Job drawing, mm, ordinate dimensions from the low corner. One solid piece. Give positions to 0.01 mm unless a question says otherwise; leave off trailing zeros. Loops run counter-clockwise (first coordinate to the right, second up) from the corner with the lowest first, then second, coordinate; pieces in that order, holes last. Notation, with made-up numbers: M 66,15 L 115,15 A21 ccw 115,22 Z; hole C 26,50.5 d8. An arc over 180 degrees is marked long. One line per question, with ' | ' between items.
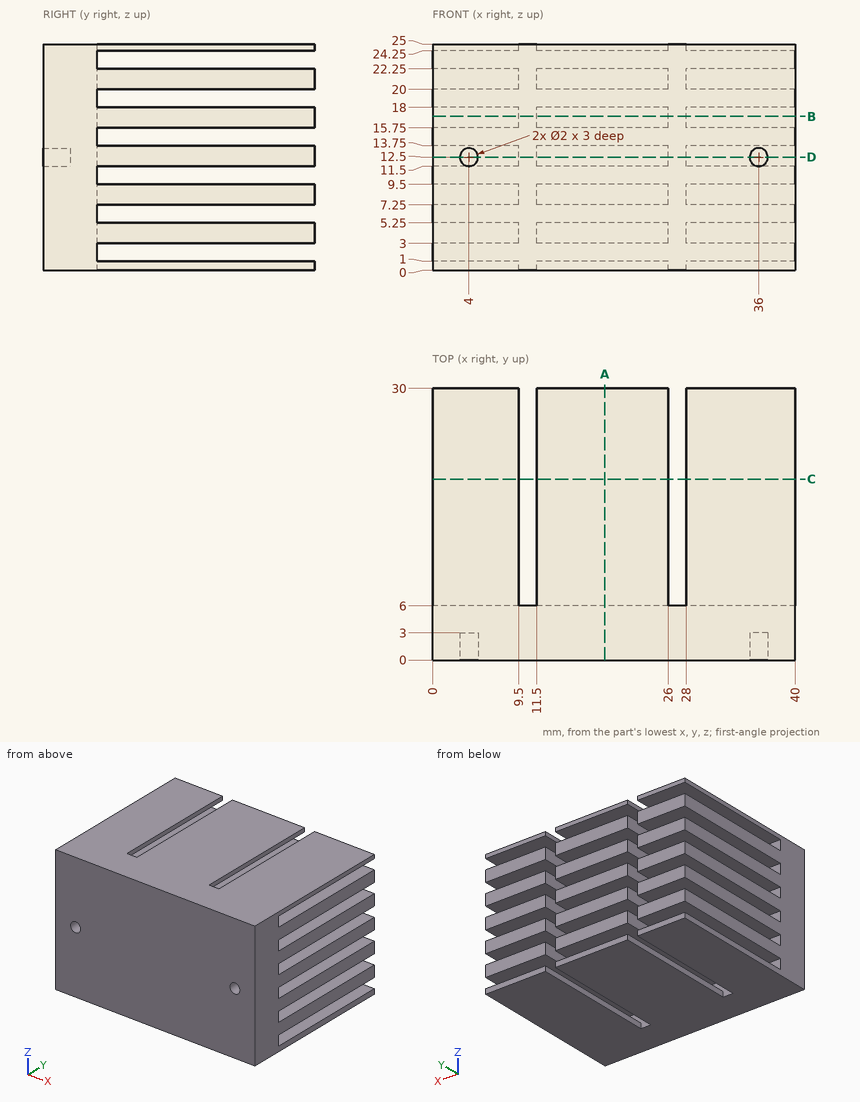
Item 1: Saw through at C-C on y = 20. State how many separate pieces and enclosed holes the cut face has, and give its area (3 significant figures).
Conclusion:
separate pieces: 21 | enclosed holes: 0 | area: 468 mm²
Item 2: Saw through at D-D on z = 12.5. Give the cut face in (x, y), and give its area (3 significant figures).
Conclusion:
outline: M 0,0 L 3,0 L 3,3 L 5,3 L 5,0 L 35,0 L 35,3 L 37,3 L 37,0 L 40,0 L 40,30 L 28,30 L 28,6 L 26,6 L 26,30 L 11.5,30 L 11.5,6 L 9.5,6 L 9.5,30 L 0,30 Z | area: 1,090 mm²
Item 3: Saw through at A-A on x = 19. Give the cut face in (y, z).
Conclusion:
outline: M 0,0 L 30,0 L 30,1 L 6,1 L 6,3 L 30,3 L 30,5.25 L 6,5.25 L 6,7.25 L 30,7.25 L 30,9.5 L 6,9.5 L 6,11.5 L 30,11.5 L 30,13.75 L 6,13.75 L 6,15.75 L 30,15.75 L 30,18 L 6,18 L 6,20 L 30,20 L 30,22.25 L 6,22.25 L 6,24.25 L 30,24.25 L 30,25 L 0,25 Z
Item 4: Drill centre lines: line 1 along X through (y, z) = (2.2, 12.5); line 2 along X through (y, z) = (9.75, 16); line 3 along Z through (x, y) = (4, 0.85). Where is each one in solid material? Low to high. Write a range as [from, to].
Conclusion:
line 1: [0, 3], [5, 35], [37, 40] | line 2: [0, 9.5], [11.5, 26], [28, 40] | line 3: [0, 11.5], [13.5, 25]
Item 5: Drop a flat-ended pin along its axis: P1, Ø6, axis at x = 14, z = 2.5, coming from the -Y side. Give the stop position or say it passes through.
Conclusion:
P1: y = 0
Item 6: Saw through at B-B on z = 17. Give the cut face in (x, y).
Conclusion:
outline: M 0,0 L 40,0 L 40,30 L 28,30 L 28,6 L 26,6 L 26,30 L 11.5,30 L 11.5,6 L 9.5,6 L 9.5,30 L 0,30 Z
